Input: part model. Units: mm. Frame: model coordinates. A direction names the side the tool comes from. Round coordinates to 2 decimals unless told otherwise and drop trailing zeros.
(1) Line query: line 1 (Z direction, x = -45.5, y = 119.5); line 2 (X direction, y = 52.5, z = -11.5); line 3 (Y direction, x = -45, z = -3). Output: solid intervals per line, ascending.
(2) First-contact query: pin 1 Ø1 at (x, y) = (-41, 12.5) entering from -Z; pin 2 Ø1 at (y, z) = (80.5, 1.5) entering from +X; pin 3 Ø5 at (x, y) = (-29.5, 22.5) entering from +Z. Flat tips, straight axial feed; report the tip coordinate or a pass-through.
(3) Access query for faces 4 (the face through (-17.085, 58.165, -18.251)), 5 (the face through (0, 62, 27)), 6 (the face through (-23.92, 110.07, -25.55)), 7 (the face through (-52, 120, -1)), 8 (the face through (49, 120, -25)). Directions: +Z, -Z, +X, -X, +Y, -Y. A direction counts if a zero-diameter tool reaches every point of the face in a straight line with its end or side. Return the directions, or none.
(4) Draft query along Y for faces 1 (the face through (52, 120, -26)), 2 (the face through (-18, 10, -18)), 3 (the face through (0.42, 57.42, -28.89)). Return one class per face: released by +Y, released by -Y, zero draft, split by the parting line, or undercut.
from build123d import *

# Parameters (mm, degrees)
SKETCH1_W           = 104
SKETCH1_H           = 104
BOSS_EXTRUDE1_DEPTH = 57.5
BOSS_EXTRUDE1_TAPER = 23
SKETCH2_R           = 25
CUT_EXTRUDE2_DEPTH  = 137.502747386
SKETCH3_R           = 35
CUT_EXTRUDE4_DEPTH  = 10
CUT_EXTRUDE5_START  = -10
SKETCH4_R           = 35
CUT_EXTRUDE5_DEPTH  = 10
SKETCH5_W           = 52
SKETCH5_H           = 52
CUT_EXTRUDE6_DEPTH  = 137.502747386
FILLET1_R           = 15
BOSS_EXTRUDE3_DEPTH = 10
FILLET2_R           = 5


with BuildPart() as part:
    # Sketch1 → Boss-Extrude1 (new body)
    with BuildSketch(Plane(origin=(0, 0, 0), x_dir=(1, 0, 0), z_dir=(0, 1, 0))):
        Rectangle(SKETCH1_W, SKETCH1_H)
    extrude(amount=BOSS_EXTRUDE1_DEPTH, taper=BOSS_EXTRUDE1_TAPER)

    # Mirror1: part across plane


with BuildPart() as part_1:
    add(part.part)
    add(part.part.mirror(Plane.ZX.offset(57.5)))

    # Sketch2 → Cut-Extrude2 (cut, through all)
    with BuildSketch(Plane(origin=(0, 115, 0), x_dir=(1, 0, 0), z_dir=(0, 1, 0))):
        with Locations(Location((0, 0, 0), (0, 0, 270))):
            Circle(SKETCH2_R)
    extrude(amount=-CUT_EXTRUDE2_DEPTH, mode=Mode.SUBTRACT)

    # Sketch3 → Cut-Extrude4 (cut)
    with BuildSketch(Plane(origin=(0, 115, 0), x_dir=(1, 0, 0), z_dir=(0, 1, 0))):
        with Locations(Location((0, 0, 0), (0, 0, 270))):
            Circle(SKETCH3_R)
    extrude(amount=-CUT_EXTRUDE4_DEPTH, mode=Mode.SUBTRACT)

    # Sketch4 → Cut-Extrude5 (cut)
    with BuildSketch(Plane.XZ.offset(CUT_EXTRUDE5_START)):
        with Locations(Location((0, 0, 0), (0, 0, 90))):
            Circle(SKETCH4_R)
    extrude(amount=CUT_EXTRUDE5_DEPTH, mode=Mode.SUBTRACT)

    # Sketch5 → Cut-Extrude6 (cut, through all)
    with BuildSketch(Plane(origin=(0, 115, 0), x_dir=(1, 0, 0), z_dir=(0, 1, 0))):
        with Locations((26, -26)):
            Rectangle(SKETCH5_W, SKETCH5_H)
    extrude(amount=-CUT_EXTRUDE6_DEPTH, mode=Mode.SUBTRACT)

    # Fillet1
    # the kernel refuses this fillet: 15 mm, written as the material it adds along each edge
    with BuildSketch(Plane(origin=(43.510503676, 57.5, -27.592698068), x_dir=(0, -0.9205048534524403, -0.3907311284892741), z_dir=(-1, 0, 0))) as fillet1_piece_1_section:
        with BuildLine():
            CenterArc((FILLET1_R * 0.42447481621, -FILLET1_R), FILLET1_R, 90, 46)
            Line((-FILLET1_R * 0.294864984129, -FILLET1_R * 0.305341629541), (0, 0))
            Line((0, 0), (FILLET1_R * 0.42447481621, 0))
        make_face()
    fillet1_piece_1 = extrude(amount=87.021007352, mode=Mode.PRIVATE)
    fillet1_piece_1 = fillet1_piece_1 - Plane(origin=(43.888103729, 57.5, -27.592698068), x_dir=(-0.9205048534524399, -0.39073112848927477, 0), z_dir=(0, 0, 1)) * Cylinder(15, 200, mode=Mode.PRIVATE)
    fillet1_piece_1 = fillet1_piece_1 - Plane(origin=(-43.888103729, 57.5, -27.592698068), x_dir=(0.9205048534524399, -0.3907311284892748, 0), z_dir=(0, 0, -1)) * Cylinder(15, 200, mode=Mode.PRIVATE)
    add(fillet1_piece_1)
    with BuildSketch(Plane(origin=(-27.592698068, 57.5, -43.510503676), x_dir=(-0.3907311284892741, -0.9205048534524403, 0), z_dir=(0, 0, 1))) as fillet1_piece_2_section:
        with BuildLine():
            CenterArc((FILLET1_R * 0.42447481621, -FILLET1_R), FILLET1_R, 90, 46)
            Line((-FILLET1_R * 0.294864984129, -FILLET1_R * 0.305341629541), (0, 0))
            Line((0, 0), (FILLET1_R * 0.42447481621, 0))
        make_face()
    fillet1_piece_2 = extrude(amount=87.021007352, mode=Mode.PRIVATE)
    fillet1_piece_2 = fillet1_piece_2 - Plane(origin=(-27.592698068, 57.5, 43.888103729), x_dir=(0, -0.39073112848927466, -0.9205048534524399), z_dir=(-1, 0, 0)) * Cylinder(15, 200, mode=Mode.PRIVATE)
    fillet1_piece_2 = fillet1_piece_2 - Plane(origin=(-27.592698068, 57.5, -43.888103729), x_dir=(0, -0.39073112848927477, 0.9205048534524399), z_dir=(1, 0, 0)) * Cylinder(15, 200, mode=Mode.PRIVATE)
    add(fillet1_piece_2)
    with BuildSketch(Plane(origin=(-43.510503676, 57.5, 27.592698068), x_dir=(0, -0.9205048534524398, 0.39073112848927505), z_dir=(1, 0, 0))) as fillet1_piece_3_section:
        with BuildLine():
            CenterArc((FILLET1_R * 0.42447481621, -FILLET1_R), FILLET1_R, 90, 46)
            Line((-FILLET1_R * 0.294864984129, -FILLET1_R * 0.305341629541), (0, 0))
            Line((0, 0), (FILLET1_R * 0.42447481621, 0))
        make_face()
    fillet1_piece_3 = extrude(amount=43.510503676, mode=Mode.PRIVATE)
    fillet1_piece_3 = fillet1_piece_3 - Plane(origin=(-43.888103729, 57.5, 27.592698068), x_dir=(0.9205048534524399, -0.3907311284892748, 0), z_dir=(0, 0, -1)) * Cylinder(15, 113, mode=Mode.PRIVATE)
    add(fillet1_piece_3)
    with BuildSketch(Plane(origin=(27.592698068, 57.5, 0), x_dir=(0.3907311284892755, -0.9205048534524396, 0), z_dir=(0, 0, -1))) as fillet1_piece_4_section:
        with BuildLine():
            CenterArc((FILLET1_R * 0.42447481621, -FILLET1_R), FILLET1_R, 90, 46)
            Line((-FILLET1_R * 0.294864984129, -FILLET1_R * 0.305341629541), (0, 0))
            Line((0, 0), (FILLET1_R * 0.42447481621, 0))
        make_face()
    fillet1_piece_4 = extrude(amount=43.510503676, mode=Mode.PRIVATE)
    fillet1_piece_4 = fillet1_piece_4 - Plane(origin=(27.592698068, 57.5, -43.888103729), x_dir=(0, -0.39073112848927477, 0.9205048534524399), z_dir=(1, 0, 0)) * Cylinder(15, 113, mode=Mode.PRIVATE)
    add(fillet1_piece_4)

    # Sketch6 → Boss-Extrude3 (add)
    with BuildSketch(Plane(origin=(0, 115, 0), x_dir=(1, 0, 0), z_dir=(0, 1, 0))):
        Polygon((49, 3), (49, 0), (52, 0), (52, 52), (-52, 52), (-52, -52), (0, -52), (0, -49), (-3, -49), (-49, -49), (-49, 49), (49, 49), align=None)
    extrude(amount=BOSS_EXTRUDE3_DEPTH)

    # Fillet2
    fillet2_edges = [part_1.edges().sort_by_distance(p)[0] for p in [
        (0, 115, -52),
        (-52, 115, 0),
        (-26, 115, 52),
        (52, 115, -26),
    ]]
    fillet(fillet2_edges, radius=FILLET2_R)


solid = part_1.part
Reported:
1. line 1: z = -52 to -49, 49 to 52
1. line 2: x = -29.75 to -22.2, 22.2 to 29.75
1. line 3: y = 0 to 16.49, 98.51 to 115
2. pin 1: stops at z = -46.91
2. pin 2: stops at x = -24.92
2. pin 3: stops at z = 43.51
3. face 4: +Y, -Y
3. face 5: +Z, +X, +Y, -Y
3. face 6: +Y
3. face 7: +Z, -Z, -X, +Y, -Y
3. face 8: +Z, +Y
4. face 1: zero draft
4. face 2: released by -Y
4. face 3: undercut
